Geometry check sheet. Reference: the model listing, model coordinates, mm. Round coordinates to 2 decimals unless told otherwise and drop trailing zeros. Write each loop counter-clockwise with the first axis right and the second up, starting at its lowest first coordinate (ties: lowest second). Pieces come first, ordered by that corner, then holes. Notation, with made-up numbers: M -7.75,88.5 L 17.25,88.5 A11 ccw 17.25,95.5 Z; hole C 50,29.25 d4. An arc over 180 degrees is marked long. One line per item, written item: value. Start each with the question number.
1. Section check A-A (z = 0). Record the boundary of the cut face in (x, y).
2. Section check D-D (x = -2.5). Record the boundary of the cut face in (y, z), and give its area (3 significant figures).
3. Depth check by flat-ended pin: P1, Ø12, axis at x = -3.5, z = -12.5, coming from the +Y side. Enter the tip coordinate at first touch or a pass-through.
4. Scan lines: probe 1 along X at (y, z) = (0.05, 2); probe 2 along Z at (x, y) = (-4.75, 0.05); probe 3 along Z at (x, y) = (10.25, 0.1). Record each from-to range of solid material in increasing order. Write a range as [from, to].
5. Section check B-B (y = 0.1). Record the boundary of the cut face in (x, z) (1 decimal), and give its area (3 significant figures).
6. Section check C-C (z = -17). Record the boundary of the cut face in (x, y).
Autodesk Inventor part; units mm, degrees
ref_plane "YZ Plane" through (0, 0, 0) normal (1, 0, 0) x (0, 1, 0)
ref_plane "XZ Plane" through (0, 0, 0) normal (0, 1, 0) x (-1, 0, 0)
ref_plane "XY Plane" through (0, 0, 0) normal (0, 0, 1) x (1, 0, 0)
sketch "Sketch1" plane through (0, 0, 0) normal (0, 1, 0) x (-1, 0, 0)
  line L0 (-7.6804, 9.5695) -> (-1.6804, 9.5695)
  line L1 (-4.6804, 5.5695) -> (-4.6804, 5.5695)
  line L2 (-0.6897, -20.436) -> (5.3214, -20.425)
  line L3 (-0.6897, -20.436) -> (-2.6847, -20.4274)
  line L4 (-3.6804, -19.4275) -> (-3.6804, 4.5695)
  line L5 (-5.6804, 4.5695) -> (-5.6804, -19.4328)
  line L6 (0.3196, 7.5695) -> (0.3196, -12.405)
  line L7 (-6.6804, -20.4328) -> (-14.6804, -20.4328)
  line L8 (-9.6804, 7.5695) -> (-9.6804, -12.4328)
  arc A0 (-7.6804, 9.5695) -> (-9.6804, 7.5695) centre (-7.6804, 7.5695) ccw
  arc A1 (0.3196, 7.5695) -> (-1.6804, 9.5695) centre (-1.6804, 7.5695) ccw
  line L9 (6.3196, -19.425) -> (6.3196, -17.4232)
  line L10 (5.3196, -16.4232) -> (1.3196, -16.4232)
  line L11 (0.3196, -15.4232) -> (0.3196, -8.8508)
  line L12 (-15.6804, -19.4328) -> (-15.6804, -17.4328)
  line L13 (-14.6804, -16.4328) -> (-10.6804, -16.4328)
  line L14 (-9.6804, -15.4328) -> (-9.6804, -12.4328)
  arc A2 (-10.6804, -16.4328) -> (-9.6804, -15.4328) centre (-10.6804, -15.4328) ccw
  arc A3 (-14.6804, -16.4328) -> (-15.6804, -17.4328) centre (-14.6804, -17.4328) ccw
  arc A4 (-15.6804, -19.4328) -> (-14.6804, -20.4328) centre (-14.6804, -19.4328) ccw
  arc A5 (-6.6804, -20.4328) -> (-5.6804, -19.4328) centre (-6.6804, -19.4328) ccw
  arc A6 (-3.6804, -19.4275) -> (-2.6847, -20.4274) centre (-2.6804, -19.4275) ccw
  arc A7 (5.3214, -20.425) -> (6.3196, -19.425) centre (5.3196, -19.425) ccw
  arc A8 (6.3196, -17.4232) -> (5.3196, -16.4232) centre (5.3196, -17.4232) ccw
  arc A9 (0.3196, -15.4232) -> (1.3196, -16.4232) centre (1.3196, -15.4232) ccw
  arc A10 (-4.6804, 5.5695) -> (-5.6804, 4.5695) centre (-4.6804, 4.5695) ccw
  arc A11 (-3.6804, 4.5695) -> (-4.6804, 5.5695) centre (-4.6804, 4.5695) ccw
  point P0 (0, 0)
  point P1 (6.3196, -20.4232)
  point P2 (-3.6804, -20.4232)
  point P3 (-15.6804, -20.4328)
  point P4 (-4.6804, 9.5695)
  point P5 (-4.6804, 5.5695)
  point P6 (2.3159, -20.4305)
  point P7 (6.3196, -16.4232)
  point P8 (-15.6804, -16.4328)
  point P9 (0.3196, -12.405)
  point P10 (-15.6804, -18.4328)
  point P11 (6.3196, -18.4241)
  dimension "d0" = 10
  dimension "d2" = 4
  dimension "d3" = 4
  dimension "d4" = 2
  dimension "d5" = 4
  dimension "d6" = 30
  dimension "d7" = 2
  dimension "d8" = 4
  dimension "d9" = 4
  dimension "d10" = 1
  dimension "d11" = 1
  dimension "d14" = 22
extrude "Extrusion1" add sketch "Sketch1" along normal blind 0.15
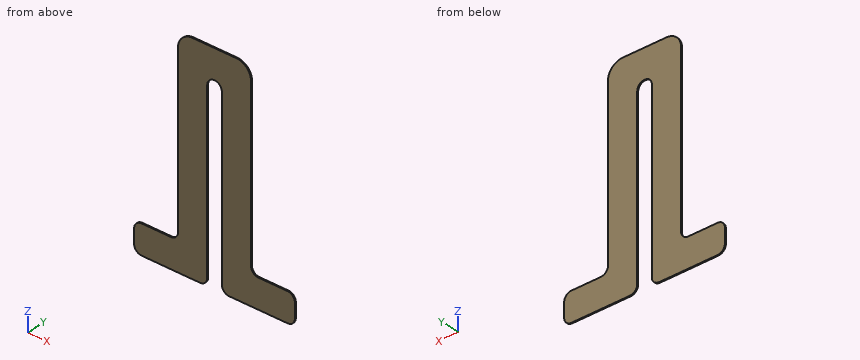
Result sheet:
1. outline: M -0.32,0 L 3.68,0 L 3.68,0.15 L -0.32,0.15 Z; M 5.68,0 L 9.68,0 L 9.68,0.15 L 5.68,0.15 Z
2. outline: M 0,-20.43 L 0.15,-20.43 L 0.15,-16.42 L 0,-16.42 Z
2. area: 0.601 mm2
3. P1: stops at y = 0.15
4. probe 1: x = [-0.32, 3.68], [5.68, 9.68]
4. probe 2: z = [-20.43, -16.42]
4. probe 3: z = [-20.43, -16.34]
5. outline: M -6.3,-19.4 A1 ccw -5.3,-20.4 L 0.7,-20.4 L 2.7,-20.4 A1 ccw 3.7,-19.4 L 3.7,4.6 A1 cw 5.7,4.6 L 5.7,-19.4 A1 ccw 6.7,-20.4 L 14.7,-20.4 A1 ccw 15.7,-19.4 L 15.7,-17.4 A1 ccw 14.7,-16.4 L 10.7,-16.4 A1 cw 9.7,-15.4 L 9.7,7.6 A2 ccw 7.7,9.6 L 1.7,9.6 A2 ccw -0.3,7.6 L -0.3,-15.4 A1 cw -1.3,-16.4 L -5.3,-16.4 A1 ccw -6.3,-17.4 Z
5. area: 294 mm2
6. outline: M -6.23,0 L 3.68,0 L 3.68,0.15 L -6.23,0.15 Z; M 5.68,0 L 15.58,0 L 15.58,0.15 L 5.68,0.15 Z
